Autodesk Inventor part; units mm, degrees
ref_plane "YZ Plane" through (0, 0, 0) normal (1, 0, 0) x (0, 1, 0)
ref_plane "XZ Plane" through (0, 0, 0) normal (0, 1, 0) x (-1, 0, 0)
ref_plane "XY Plane" through (0, 0, 0) normal (0, 0, 1) x (1, 0, 0)
sketch "スケッチ1" plane through (0, 0, 0) normal (0, 0, 1) x (1, 0, 0)
  circle A0 centre (0, 0) radius 1.85
  dimension "d0" = 3.7
extrude "押し出し1" add sketch "スケッチ1" along normal blind 2
sketch "スケッチ2" plane through (0, 0, 0) normal (0, 0, -1) x (-1, 0, 0)
  circle A0 centre (0, 0) radius 1
  dimension "d3" = 2
extrude "押し出し2" add sketch "スケッチ2" along normal blind 8
thread "ねじ1"
chamfer "面取り1" distance 0.2 angle 45 1 edges at (-1.85, 0, 2)
properties part number "M2×8" material "ステンレス鋼"
Here's how the part is built. I have some questions about the finished solid (model axes, mm). A direction names the side the tool comes from. Round coordinates to 2 decimals unless told otherwise and drop trailing zeros. Write each loop counter-clockwise with the first axis right and the second up, starting at its lowest first coordinate (ties: lowest second). Pieces come first, ordered by that corner, then holes.
Q1. If we section it at A-A on y = 0: Write out the boundary of the cut face in (x, z).
Q2. Will this pin go through, and if not, where does the flat tip stop? P1, Ø1, axis at y = 0, z = -5, coming from the +X side.
Q3. Which directions (+Z, -Z, +X, -X, +Y, -Y) give clear straight access to the entire face, cutting with the end or side of a thin tool? Please do faces 1 (the flat face through (1, -1, 0)), 2 (the flat face through (0, 0, -8)).
Q4. If we section it at C-C on z = -4.5: Write out the boundary of the cut face in (x, y).
Q5. Please list where these lines run through material, in increasing order: probe 1 along Z at (x, y) = (-0.6, -1.4); probe 2 along X at (y, z) = (0.05, -7); probe 3 along X at (y, z) = (-0.85, -3.5).
Answer below:
1. outline: (-1.85, 0) - (-1, 0) - (-1, -8) - (1, -8) - (1, 0) - (1.85, 0) - (1.85, 1.8) - (1.65, 2) - (-1.65, 2) - (-1.85, 1.8) - close
2. P1: stops at x = 1
3. face 1: -Z
3. face 2: -Z, +X, -X, +Y, -Y
4. outline: circle Ø2 at (0, 0)
5. probe 1: z = 0 to 2
5. probe 2: x = -1 to 1
5. probe 3: x = -0.53 to 0.53
